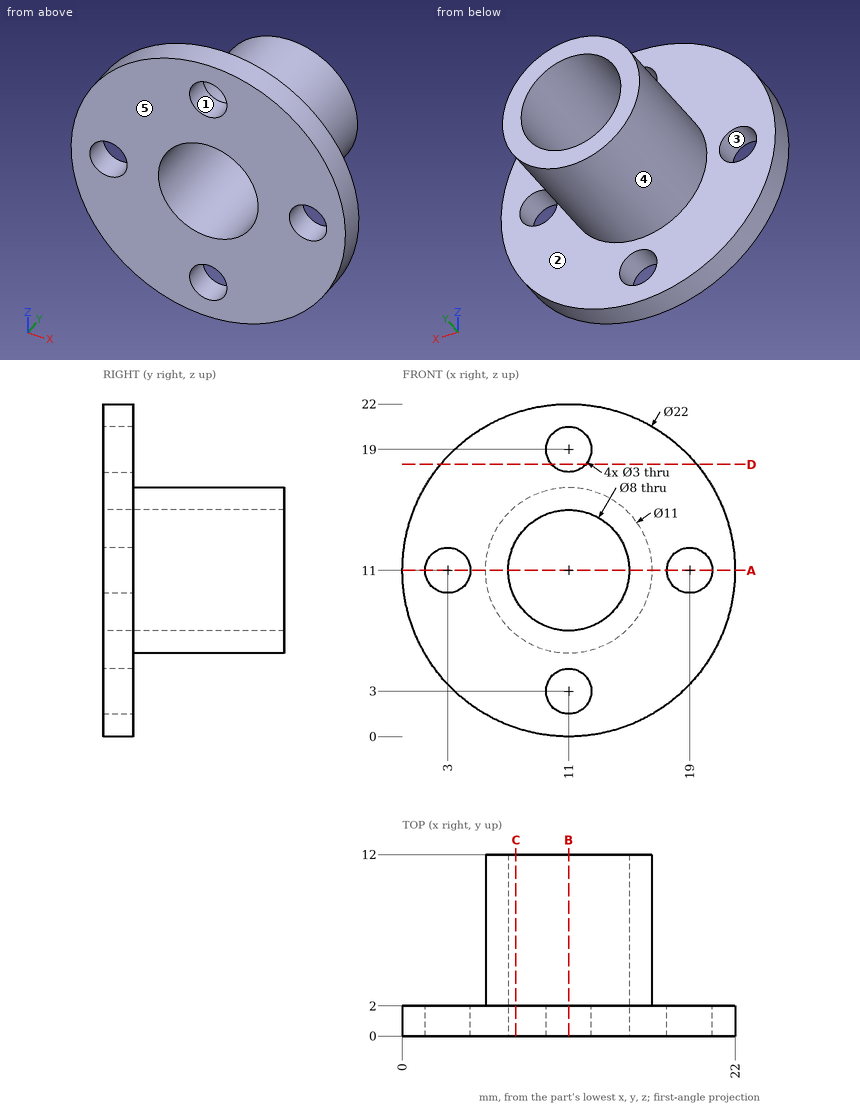
Drawing for the job (mm, zero at the part's lowest x, y, z). A direction names the side the tool comes from. Give positions to 0.01 mm unless a question says otherwise; leave off trailing zeros. Write each loop counter-clockwise with the first axis right and the second up, starting at its lowest first coordinate (ties: lowest second). Pieces come first, ordered by that corner, then holes. Notation, with made-up numbers: M 14.25,-21.75 L 28.25,-21.75 A18 ccw 28.25,-0.75 Z; hole C 71.5,14 d7. An arc over 180 degrees is marked long. Return JSON: item names as keys, results as strings. Group by question number.
(1) Band-saw the part on A-A (z = 11). Give the cut face in (x, y).
(2) Band-saw the part on C-C (x = 7.5). Give the cut face in (y, z).
(3) Mould opens along Z. For the marked faces 3, 4 and 5 say: pulls with the +Z half, pulls with the -Z half, needs draft (parallel to the pull), parting line crosses it, or undercut.
(4) Band-saw the part on D-D (z = 18). Give the cut face in (x, y), and give its area (3 significant figures).
(5) Drill centre lines: L1, parallel to X at y = 0.8, z = 11; L2, parallel to X at y = 2.5, z = 11; L3, parallel to Y at x = 4.75, z = 15.5. Where is each one in solid material? Low to high. Write a range as [from, to].
(6) Band-saw the part on B-B (x = 11). Give the cut face in (y, z).
(7) 3-axis set-ups, long thin cutter, end or side, ignore diameter. For the marked faces 1 and 2: which of +Z, -Z, +X, -X, +Y, -Y reach the whole face in a straight line?
(8) Flat gauge pins, fed straight in: pin 1 Ø8 at (x, z) = (16.5, 19) entering from +Y; pin 2 Ø3 at (x, y) = (14.5, 2) entering from -Z; pin 3 Ø5 at (y, z) = (10.5, 13) entering from +X. Where does each tip first touch, or does it go through?
Entries:
{
 "1": {"outline": "M 0,0 L 1.5,0 L 1.5,2 L 0,2 Z; M 4.5,0 L 7,0 L 7,12 L 5.5,12 L 5.5,2 L 4.5,2 Z; M 15,0 L 17.5,0 L 17.5,2 L 16.5,2 L 16.5,12 L 15,12 Z; M 20.5,0 L 22,0 L 22,2 L 20.5,2 Z"},
 "2": {"outline": "M 0,0.57 L 2,0.57 L 2,6.76 L 12,6.76 L 12,9.06 L 0,9.06 Z; M 0,12.94 L 12,12.94 L 12,15.24 L 2,15.24 L 2,21.43 L 0,21.43 Z"},
 "3": {"face 3": "undercut", "face 4": "parting line crosses it", "face 5": "needs draft"},
 "4": {"outline": "M 2.51,0 L 9.88,0 L 9.88,2 L 2.51,2 Z; M 12.12,0 L 19.49,0 L 19.49,2 L 12.12,2 Z", "area": "29.5 mm^2"},
 "5": {"L1": "x = [0, 1.5], [4.5, 7], [15, 17.5], [20.5, 22]", "L2": "x = [5.5, 7], [15, 16.5]", "L3": "y = [0, 2]"},
 "6": {"outline": "M 0,0 L 2,0 L 2,1.5 L 0,1.5 Z; M 0,4.5 L 2,4.5 L 2,5.5 L 12,5.5 L 12,7 L 0,7 Z; M 0,15 L 12,15 L 12,16.5 L 2,16.5 L 2,17.5 L 0,17.5 Z; M 0,20.5 L 2,20.5 L 2,22 L 0,22 Z"},
 "7": {"face 1": "+Y, -Y", "face 2": "+Y"},
 "8": {"pin 1": "stops at y = 2", "pin 2": "stops at z = 0.18", "pin 3": "stops at x = 16.5"}
}
